The listing builds one solid part. Answer for the finished solid, in the listing's coordinates (mm). A direction names the side the tool comes from. Give positions to 0.01 mm unless a question says otherwise; leave off trailing zeros. Write each loop counter-clockwise with the first axis right and the second up, starting at its lowest first coordinate (ties: lowest second). Pieces come first, ordered by that corner, then holes. Notation, with made-up numbers: (67, 71.25) -> (110, 71.25) arc R3 cw to (110, 76.25) -> close; hole circle Ø2 at (12, 73). An arc over 180 degrees is marked (long way). Put each result on its own line as item: value. Start each with the question number.
1) A cutting plane is placed at A-A (x = 0). Write down the section's boundary in (y, z).
2) For faces 4 (the cylindrical face through (-3.967, 4.695, -0.881)), 5 (the cylindrical face through (-2.03, 1.93, 1.05)), determine the directions among +Z, -Z, +X, -X, +Y, -Y from which every point of the face is accessible in a straight line to the end or side of a thin tool.
3) Find the intervals of material crossed by line 1 along X through (y, z) = (2.65, 0); line 2 along Y through (x, z) = (1.75, -3.5); line 3 along X through (y, z) = (3.25, -1.75), in increasing order. Write a range as from..to.
4) For a pull along Z with two mould halves and no side action, classify faces 1 (the flat face through (-2, 3.81, 2)), 2 (the flat face through (-5, 6.35, 2)), 3 (the cylindrical face through (-3.86, 3.14, -5.04)) as released by +Z, released by -Z, zero draft, split by the parting line, or undercut.
5) A cutting plane is placed at D-D (y = 1). Write down the section's boundary in (x, z), then the cut area to 3 significant figures.
6) A cutting plane is placed at B-B (z = 0). Write down the section's boundary in (x, y).
7) A flat-ended cylindrical pin translates along its axis: pin 1 Ø2 at (y, z) = (1, -3.5) entering from +X. Find the tip coordinate at first contact, or state that the pin passes through.
8) A cutting plane is placed at C-C (y = 4). Write down the section's boundary in (x, z), then the cut area to 3 significant figures.
from build123d import *

# Parameters (mm, degrees)
SKETCH1_R           = 6.35
BOSS_EXTRUDE1_DEPTH = 6.35
SKETCH2_R           = 2.286
CUT_EXTRUDE1_DEPTH  = 11.998522628
SKETCH3_R           = 4.064
CUT_EXTRUDE2_DEPTH  = 2.54
FILLET1_R           = 0.79375


with BuildPart() as part:
    # Sketch1 → Boss-Extrude1 (new body)
    with BuildSketch(Plane(origin=(0, 0, 0), x_dir=(1, 0, 0), z_dir=(0, 1, 0))):
        with Locations(Location((0, 0, 0), (0, 0, 270))):
            Circle(SKETCH1_R)
    extrude(amount=BOSS_EXTRUDE1_DEPTH)

    # Sketch2 → Cut-Extrude1 (cut, through all)
    with BuildSketch(Plane(origin=(0, 6.35, 0), x_dir=(1, 0, 0), z_dir=(0, 1, 0))):
        with Locations(Location((0, 0, 0), (0, 0, 270))):
            Circle(SKETCH2_R)
    extrude(amount=-CUT_EXTRUDE1_DEPTH, mode=Mode.SUBTRACT)

    # Sketch3 → Cut-Extrude2 (cut)
    with BuildSketch(Plane(origin=(0, 6.35, 0), x_dir=(1, 0, 0), z_dir=(0, 1, 0))):
        with Locations(Location((0, 0, 0), (0, 0, 270))):
            Circle(SKETCH3_R)
    extrude(amount=-CUT_EXTRUDE2_DEPTH, mode=Mode.SUBTRACT)

    # Fillet1
    fillet1_edges = [part.edges().sort_by_distance(p)[0] for p in [
        (0, 6.35, -4.064),
        (0, 0, -6.35),
        (0, 6.35, -6.35),
    ]]
    fillet(fillet1_edges, radius=FILLET1_R)


solid = part.part
Reply:
1. outline: (0, -5.56) arc R0.79 ccw to (0.79, -6.35) -> (5.56, -6.35) arc R0.79 ccw to (6.35, -5.56) -> (6.35, -4.86) arc R0.79 ccw to (5.56, -4.06) -> (3.81, -4.06) -> (3.81, -2.29) -> (0, -2.29) -> close; (0, 2.29) -> (3.81, 2.29) -> (3.81, 4.06) -> (5.56, 4.06) arc R0.79 ccw to (6.35, 4.86) -> (6.35, 5.56) arc R0.79 ccw to (5.56, 6.35) -> (0.79, 6.35) arc R0.79 ccw to (0, 5.56) -> close
2. face 4: +Y
2. face 5: +Y, -Y
3. line 1: x = -6.35..-2.29, 2.29..6.35
3. line 2: y = 0..3.81
3. line 3: x = -6.1..-1.47, 1.47..6.1
4. face 1: undercut
4. face 2: zero draft
4. face 3: split by the parting line
5. outline: circle Ø12.7 at (0, 0); hole circle Ø4.57 at (0, 0)
5. area: 110 mm2
6. outline: (-6.35, 0.79) arc R0.79 ccw to (-5.56, 0) -> (-2.29, 0) -> (-2.29, 3.81) -> (-4.06, 3.81) -> (-4.06, 5.56) arc R0.79 ccw to (-4.86, 6.35) -> (-5.56, 6.35) arc R0.79 ccw to (-6.35, 5.56) -> close; (2.29, 0) -> (5.56, 0) arc R0.79 ccw to (6.35, 0.79) -> (6.35, 5.56) arc R0.79 ccw to (5.56, 6.35) -> (4.86, 6.35) arc R0.79 ccw to (4.06, 5.56) -> (4.06, 3.81) -> (2.29, 3.81) -> close
7. pin 1: stops at x = 5.84
8. outline: circle Ø12.7 at (0, 0); hole circle Ø8.13 at (0, 0)
8. area: 74.8 mm2
